Verification items for the finished model (mm, model axes). A direction names the side the tool comes from. Coordinates: 2 decimals unless noted, no trailing zeros. Write each loop counter-clockwise with the first axis right and the second up, starting at its lowest first coordinate (ties: lowest second). Pieces come first, ordered by that corner, then holes. Notation, with made-up numbers: (9.5, -18.5) -> (16.5, -18.5) arc R13 ccw to (16.5, 1.5) -> close; hole circle Ø4 at (11.25, -29.75). An arc over 180 degrees is marked (long way). Answer in a Markdown table with one row per item.
```python
from build123d import *

# Parameters (mm, degrees)
SKETCH1_W           = 300
SKETCH1_H           = 150
BOSS_EXTRUDE1_DEPTH = 20
SKETCH2_W           = 80.25
SKETCH2_H           = 30
CUT_EXTRUDE1_DEPTH  = 15
SKETCH3_R           = 10
BOSS_EXTRUDE2_DEPTH = 20


with BuildPart() as part:
    # Sketch1 → Boss-Extrude1 (new body)
    with BuildSketch(Plane.XY):
        Rectangle(SKETCH1_W, SKETCH1_H)
    extrude(amount=BOSS_EXTRUDE1_DEPTH)

    # Sketch2 → Cut-Extrude1 (cut)
    with BuildSketch(Plane(origin=(0, 0, 0), x_dir=(-1, 0, 0), z_dir=(0, 0, -1))):
        with Locations((50.125, 0)):
            Rectangle(SKETCH2_W, SKETCH2_H)
    extrude(amount=-CUT_EXTRUDE1_DEPTH, mode=Mode.SUBTRACT)

    # Sketch3 → Boss-Extrude2 (add)
    with BuildSketch(Plane(origin=(0, 30, 0), x_dir=(1, 0, 0), z_dir=(0, 1, 0))):
        with BuildLine():
            Line((56.38, 0), (56.38, 12.86))
            ThreePointArc((56.38, 12.86), (76.38, 32.86), (96.38, 12.86))
            Line((96.38, 12.86), (96.38, 0))
            Line((96.38, 0), (56.38, 0))
        make_face()
        with Locations((76.38, 12.86)):
            Circle(SKETCH3_R, mode=Mode.SUBTRACT)
    extrude(amount=-BOSS_EXTRUDE2_DEPTH)


solid = part.part
```
1. Access from +Z, -Z, +X, -X, +Y, -Y to the whole of each face (thin tool, end or side, straight path). Record for faces 1 (the face through (56.38, 20, -6)), 2 (the face through (96.38, 20, -7)), 3 (the face through (77, 30, -24)), 4 (the face through (-50, 0, 15)), 5 (the face through (-2, -75, 10)).
Findings below:
| item | result |
|---|---|
| face 1 | -Z, -X, +Y, -Y |
| face 2 | -Z, +X, +Y, -Y |
| face 3 | -Z, +X, -X, +Y |
| face 4 | -Z |
| face 5 | +Z, -Z, +X, -X, -Y |
2. Go/stop test with flat-tipped pins: pin 1 (5 mm diameter, centred on x = 80.5, y = 22.5, fed in from -Z); pin 2 (8 mm diameter, centred on x = -37, y = 56.5, fed in from -Z); pin 3 (4 mm diameter, centred on y = 17, z = -8.5, fed in from -X); pin 4 (8 mm diameter, centred on y = -21.5, z = -7.5, fed in from +X). Record where each tip stops, or that it passes through.
Findings below:
| item | result |
|---|---|
| pin 1 | stops at z = -32.79 |
| pin 2 | stops at z = 0 |
| pin 3 | stops at x = 56.38 |
| pin 4 | passes through |
3. Sectioned sample at A-A, the plane x = 76.38. Record the cut outline in (y, z).
Findings below:
| item | result |
|---|---|
| outline | (-75, 0) -> (10, 0) -> (10, -2.86) -> (30, -2.86) -> (30, 0) -> (75, 0) -> (75, 20) -> (-75, 20) -> close; (10, -32.86) -> (30, -32.86) -> (30, -22.86) -> (10, -22.86) -> close |
4. Sectioned sample at D-D, the plane y = 65. Record the cut outline in (x, z).
Findings below:
| item | result |
|---|---|
| outline | (-150, 0) -> (150, 0) -> (150, 20) -> (-150, 20) -> close |
5. Sectioned sample at B-B, the plane z = 3.5. Record the cut outline in (x, y), and give its area (3 significant figures).
Findings below:
| item | result |
|---|---|
| outline | (-150, -75) -> (150, -75) -> (150, 75) -> (-150, 75) -> close; hole (-90.25, -15) -> (-10, -15) -> (-10, 15) -> (-90.25, 15) -> close |
| area | 42,600 mm² |
6. Release check for a two-part mould opening along X. For faces 6 (the face through (77, 10, -24)), 7 (the face through (-10, 0, 7)), 8 (the face through (150, -1, 10)) record: released by +X, released by -X, zero draft, split by the parting line, or undercut.
Findings below:
| item | result |
|---|---|
| face 6 | zero draft |
| face 7 | undercut |
| face 8 | released by +X |
7. Sectioned sample at C-C, the plane x = -84. Record the cut outline in (y, z).
Findings below:
| item | result |
|---|---|
| outline | (-75, 0) -> (-15, 0) -> (-15, 15) -> (15, 15) -> (15, 0) -> (75, 0) -> (75, 20) -> (-75, 20) -> close |
8. Material ranges on probe 1 along X at (y, z) = (15, -12.86); probe 2 along Z at (x, y) = (76, 23); probe 3 along Y at (x, z) = (-38.5, 12.5), recorded low to high. Write a range as from..to.
Findings below:
| item | result |
|---|---|
| probe 1 | x = 56.38..66.38, 86.38..96.38 |
| probe 2 | z = -32.86..-22.85, -2.87..20 |
| probe 3 | y = -75..-15, 15..75 |
